```python
from build123d import *

# Parameters (mm, degrees)
F0_W      = 38.1
F0_H      = 38.1
F1_DEPTH  = 38.1
F6_DEPTH  = 38.1
F8_DEPTH  = 38.1
F10_DEPTH = 38.1


with BuildPart() as f1:
    # F0 (on Front) → F1 (new body)
    with BuildSketch(Plane.XZ):
        with Locations((19.05, 19.05)):
            Rectangle(F0_W, F0_H)
    extrude(amount=F1_DEPTH)

    # F5 (on offset) → F6 (cut)
    with BuildSketch(Plane.YZ.offset(38.1)):
        Polygon((-6.35, 0), (0, 0), (0, 38.1), align=None)
        Polygon((-25.4, 0), (-12.7, 0), (-19.05, 15.875), align=None)
        Polygon((-31.75, 0), (-38.1, 38.1), (-38.1, 0), align=None)
        Polygon((-11.43, 15.875), (-6.35, 38.1), (-31.75, 38.1), (-26.67, 15.875), (-21.59, 28.575), (-16.51, 28.575), align=None)
    extrude(amount=-F6_DEPTH, mode=Mode.SUBTRACT)

    # F7 (on offset) → F8 (cut)
    with BuildSketch(Plane.XZ.offset(38.1)):
        Polygon((25.4, 38.1), (12.7, 38.1), (19.05, 22.225), align=None)
        Polygon((38.1, 38.1), (31.75, 38.1), (38.1, 0), align=None)
        Polygon((11.43, 22.225), (6.35, 0), (31.75, 0), (26.67, 22.225), (21.59, 9.525), (16.51, 9.525), align=None)
        Polygon((6.35, 38.1), (0, 38.1), (0, 0), align=None)
    extrude(amount=-F8_DEPTH, mode=Mode.SUBTRACT)

    # F9 (on offset) → F10 (cut)
    with BuildSketch(Plane.XY.offset(38.1)):
        Polygon((38.1, -15.24), (38.1, -7.485609), (12.7, -7.62), (12.7, -15.24), align=None)
        Polygon((25.4, -22.86), (0, -22.86), (0, -30.480013), (25.4, -30.618137), align=None)
    extrude(amount=-F10_DEPTH, mode=Mode.SUBTRACT)


solid = f1.part
```
Source: CAD feature listing. Evaluate the final solid. Frame: model axes, mm. A direction names the side the tool comes from. Coordinates: 2 decimals unless noted, no trailing zeros. Order: outer loops, then holes, each group sorted by start corner. A loop starts at its lowest first (then second) coordinate and runs counter-clockwise, first axis right, second up. Notation, with made-up numbers: (-14, 3.25) - (-7, 3.25) arc R25 cw to (-7, 27.25) - close; hole circle Ø3 at (-24.5, 60). An arc over 180 degrees is marked (long way). One line per item, written item: value.
1) Ray query, line 1 (Y direction, x = 30.5, z = 14); line 2 (Y direction, x = 25, z = 28.5); line 3 (Y direction, x = 12, z = 35.5). Return the intervals inside material, ascending. Write a range as [from, to].
Computed values:
line 1: y = [-34.08, -19.8], [-18.3, -15.24], [-7.53, -4.02]
line 2: y = [-36.5, -30.62], [-21.62, -16.48], [-7.55, -1.6]
line 3: y = [-37.67, -31.16], [-6.94, -0.43]
2) Cut plane B-B on z = 27. Output: boundary loops of the cut face in (x, y).
Computed values:
outline: (4.5, -36.25) - (17.14, -36.25) - (17.14, -30.57) - (4.5, -30.5) - close; (4.5, -22.22) - (17.14, -22.22) - (17.14, -15.88) - (4.5, -15.88) - close; (4.5, -8.89) - (12.7, -8.89) - (12.7, -7.62) - (17.14, -7.6) - (17.14, -1.85) - (4.5, -1.85) - close; (20.96, -36.25) - (33.6, -36.25) - (33.6, -29.21) - (25.4, -29.21) - (25.4, -30.62) - (20.96, -30.59) - close; (20.96, -22.22) - (33.6, -22.22) - (33.6, -15.88) - (20.96, -15.88) - close; (20.96, -7.58) - (33.6, -7.51) - (33.6, -1.85) - (20.96, -1.85) - close
3) Contact query for flat-ended pins moving along their axis: pin 1 (1 mm diameter, centred on y = -29.5, z = 28, fed in from -X); pin 2 (1 mm diameter, centred on y = -16.5, z = 25.5, fed in from -X); pin 3 (9.5 mm diameter, centred on x = 23, z = 20.5, fed in from +Y); pin 4 (1 mm diameter, centred on x = 18.5, z = 7.5, fed in from -Y). Output: stop coordinate, or through.
Computed values:
pin 1: stops at x = 25.4
pin 2: stops at x = 4.17
pin 3: stops at y = -2.14
pin 4: passes through
4) Cut plane A-A on y = -1.5. Output: boundary loops of the cut face in (x, z), plus the area to 3 significant figures.
Computed values:
outline: (4.85, 29.1) - (16.3, 29.1) - (12.7, 38.1) - (6.35, 38.1) - close; (21.8, 29.1) - (33.25, 29.1) - (31.75, 38.1) - (25.4, 38.1) - close
area: 160 mm^2
5) Cut plane C-C on z = 4. Output: boundary loops of the cut face in (x, y), plus the area to 3 significant figures.
Computed values:
outline: (0.67, -32.42) - (7.26, -32.42) - (7.26, -30.52) - (0.67, -30.48) - close; (0.67, -14.3) - (7.26, -14.3) - (7.26, -5.68) - (0.67, -5.68) - close; (30.84, -32.42) - (37.43, -32.42) - (37.43, -23.8) - (30.84, -23.8) - close; (30.84, -7.52) - (37.43, -7.49) - (37.43, -5.68) - (30.84, -5.68) - close
area: 138 mm^2
6) Cut plane D-D on x = 26. Output: boundary loops of the cut face in (y, z) (3 decimals), plus the area to 3 significant figures.
Computed values:
outline: (-38.1, 38.1) - (-35.175, 20.55) - (-27.739, 20.55) - (-31.75, 38.1) - close; (-24.8, 20.55) - (-15.24, 20.55) - (-15.24, 25.4) - (-16.51, 28.575) - (-21.59, 28.575) - close; (-7.55, 20.55) - (-2.925, 20.55) - (0, 38.1) - (-6.35, 38.1) - (-7.55, 32.852) - close
area: 286 mm^2
7) Reachability of faces 4 (the face through (22.2, -33.6, 30.1)), 5 (the face through (9.49, -12.89, 13.74)), 6 (the face through (8.6, -14, 22.3)), 7 (the face through (25.4, -24, 21)), 8 (the face through (29, -3, 38.1)) from +Z, -Z, +X, -X, +Y, -Y: full face, straight path, thin tool, end or side. Return the list, or none.
Computed values:
face 4: +Z, +Y, -Y
face 5: -Z, +Y, -Y
face 6: +Z, +X, -X
face 7: +Z, -Z, -X
face 8: +Z, +X, -X, +Y, -Y
8) Mould query, pull axis Y, two halves, no side actions, for faces 1 (the face through (11.1, -22.23, 26.97)), 2 (the face through (22.2, -4.7, 30.1)), 3 (the face through (19.32, -3.13, 19.32)). Classes: released by +Y, released by -Y, zero draft, split by the parting line, or undercut.
Computed values:
face 1: undercut
face 2: zero draft
face 3: released by +Y
